Part model, mm, in its own coordinate system. Give positions to 0.01 mm unless a question says otherwise; leave off trailing zeros. Loops run counter-clockwise (first coordinate to the right, second up) from the corner with the lowest first, then second, coordinate; pieces in that order, holes last. Notation, with made-up numbers: M 17,50.25 L 69,50.25 A30 cw 69,77.25 Z; hole C 61.25,-39.75 d3. An arc over 180 degrees is marked long. Put each result on its own line as item: value. Start each with the question number.
```python
from build123d import *

# Parameters (mm, degrees)
ARRAY_X_COUNT = 2
ARRAY_X_PITCH = 12
ARRAY_Y_COUNT = 2
ARRAY_Y_PITCH = 12
BOX001_W      = 1
BOX001_H      = 18
BOX001_DEPTH  = 10
BOX_W         = 40
BOX_H         = 20
BOX_DEPTH     = 10


with BuildPart() as esfera004:
    # Sphere004 → Sphere004 (revolve)
    with BuildSketch(Plane(origin=(36, 16, 10), x_dir=(1, 0, 0), z_dir=(0, -1, 0))):
        with BuildLine():
            ThreePointArc((0, -2), (2, 0), (0, 2))
            Line((0, 2), (0, -2))
        make_face()
    revolve(axis=Axis((36, 16, 10), (0, 0, 1)))


with BuildPart() as esfera003:
    # Sphere003 → Sphere003 (revolve)
    with BuildSketch(Plane(origin=(30, 10, 10), x_dir=(1, 0, 0), z_dir=(0, -1, 0))):
        with BuildLine():
            ThreePointArc((0, -2), (2, 0), (0, 2))
            Line((0, 2), (0, -2))
        make_face()
    revolve(axis=Axis((30, 10, 10), (0, 0, 1)))


with BuildPart() as esfera002:
    # Sphere002 → Sphere002 (revolve)
    with BuildSketch(Plane(origin=(24, 4, 10), x_dir=(1, 0, 0), z_dir=(0, -1, 0))):
        with BuildLine():
            ThreePointArc((0, -2), (2, 0), (0, 2))
            Line((0, 2), (0, -2))
        make_face()
    revolve(axis=Axis((24, 4, 10), (0, 0, 1)))


with BuildPart() as esfera001:
    # Sphere001 → Sphere001 (revolve)
    with BuildSketch(Plane(origin=(10, 10, 10), x_dir=(1, 0, 0), z_dir=(0, -1, 0))):
        with BuildLine():
            ThreePointArc((0, -2), (2, 0), (0, 2))
            Line((0, 2), (0, -2))
        make_face()
    revolve(axis=Axis((10, 10, 10), (0, 0, 1)))


with BuildPart() as array:
    # Sphere → Sphere (revolve)
    with BuildSketch(Plane(origin=(4, 4, 10), x_dir=(1, 0, 0), z_dir=(0, -1, 0))):
        with BuildLine():
            ThreePointArc((0, -2), (2, 0), (0, 2))
            Line((0, 2), (0, -2))
        make_face()
    revolve(axis=Axis((4, 4, 10), (0, 0, 1)))

    # Array X: Array ×2


with BuildPart() as array_1:
    add(array.part)
    with Locations(*[(i * ARRAY_X_PITCH, 0, 0) for i in range(1, ARRAY_X_COUNT)]):
        add(array.part)

    # Array Y: Array ×2


with BuildPart() as array_2:
    add(array_1.part)
    with Locations(*[(0, i * ARRAY_Y_PITCH, 0) for i in range(1, ARRAY_Y_COUNT)]):
        add(array_1.part)


with BuildPart() as obj1:
    # Box001 → Box001 (new body)
    with BuildSketch(Plane(origin=(19.5, 1, 8), x_dir=(1, 0, 0), z_dir=(0, 0, 1))):
        with Locations((0.5, 9)):
            Rectangle(BOX001_W, BOX001_H)
    extrude(amount=BOX001_DEPTH)


with BuildPart() as cut005:
    # Box → Box (new body)
    with BuildSketch(Plane.XY):
        with Locations((20, 10)):
            Rectangle(BOX_W, BOX_H)
    extrude(amount=BOX_DEPTH)

    # Cut: cut obj1
    add(obj1.part, mode=Mode.SUBTRACT)

    # Cut001: cut Array
    add(array_2.part, mode=Mode.SUBTRACT)

    # Cut002: cut Esfera001
    add(esfera001.part, mode=Mode.SUBTRACT)

    # Cut003: cut Esfera002
    add(esfera002.part, mode=Mode.SUBTRACT)

    # Cut004: cut Esfera003
    add(esfera003.part, mode=Mode.SUBTRACT)

    # Cut005: cut Esfera004
    add(esfera004.part, mode=Mode.SUBTRACT)


solid = cut005.part
```
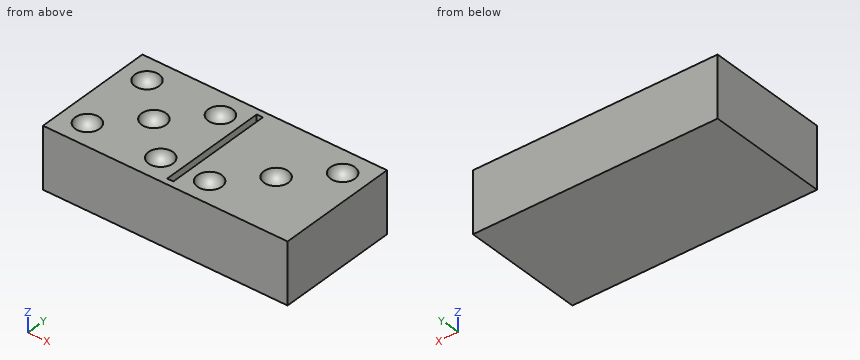
1) Pin check, flat tip, straight feed: pin 1 Ø0.5 at (x, y) = (20, 9) entering from +Z. Stop position of the tip, or through.
2) Band-saw the part on B-B on z = 8.5. State how many separate pieces and enclosed holes the cut face has, then the cut area to 3 significant figures.
3) Wall check: L1, parallel to Y at x = 23, z = 9.5; L2, parallel to Y at x = 30, z = 8.5; L3, parallel to Z at x = 16, y = 4.25. Give the ranges that are in metal, low to high.
4) Band-saw the part on C-C on x = 36.5. Give the cut face in (y, z).
5) Band-saw the part on D-D on y = 11.5. Give the cut face in (x, z).
6) Band-saw the part on A-A on y = 15.25. Give the cut face in (x, z).
Evaluation:
1. pin 1: z = 8
2. separate pieces: 1
2. enclosed holes: 9
2. area: 738 mm2
3. L1: 0 to 2.34, 5.66 to 20
3. L2: 0 to 8.68, 11.32 to 20
3. L3: 0 to 8.02
4. outline: M 0,0 L 20,0 L 20,10 L 17.94,10 A1.94 cw 14.06,10 L 0,10 Z
5. outline: M 0,0 L 40,0 L 40,10 L 31.32,10 A1.32 cw 28.68,10 L 20.5,10 L 20.5,8 L 19.5,8 L 19.5,10 L 11.32,10 A1.32 cw 8.68,10 L 0,10 Z
6. outline: M 0,0 L 40,0 L 40,10 L 37.85,10 A1.85 cw 34.15,10 L 20.5,10 L 20.5,8 L 19.5,8 L 19.5,10 L 17.85,10 A1.85 cw 14.15,10 L 5.85,10 A1.85 cw 2.15,10 L 0,10 Z
